from build123d import *

# Parameters (mm, degrees)
SKETCH1_R                = 2
BOSS_EXTRUDE2_DEPTH      = 5
BOSS_EXTRUDE3_DEPTH      = 9
BOSS_EXTRUDE3_DEPTH_BACK = 14
SKETCH3_W                = 35
SKETCH3_H                = 50
SKETCH4_W                = 13
SKETCH4_H                = 40
CUT_EXTRUDE1_DEPTH       = 194.703381488
SKETCH5_R                = 4.35
CUT_EXTRUDE2_DEPTH       = 194.053917795
CUT_EXTRUDE3_DEPTH       = 193.189529309
FILLET14_R               = 15
FILLET15_R               = 15
FILLET16_R               = 15
FILLET17_R               = 15
FILLET18_R               = 5
FILLET19_R               = 5
FILLET20_R               = 5
FILLET21_R               = 5
FILLET22_R               = 3
FILLET23_R               = 3
FILLET24_R               = 3
FILLET25_R               = 3
SKETCH7_R                = 4
CUT_EXTRUDE4_DEPTH       = 193.189529428


with BuildPart() as part:
    # Sketch1 → Boss-Extrude2 (new body)
    with BuildSketch(Plane.XY):
        with BuildLine():
            Line((-9.685672515, -15), (-9.685672515, 190))
            Line((-9.685672515, 190), (25.314327485, 190))
            Line((25.314327485, 190), (25.314327485, -15))
            ThreePointArc((25.314327485, -15), (7.814327485, -32.5), (-9.685672515, -15))
        make_face()
        with Locations((19.814327485, -15)):
            Circle(SKETCH1_R, mode=Mode.SUBTRACT)
        with Locations((7.814327485, -27)):
            Circle(SKETCH1_R, mode=Mode.SUBTRACT)
        with Locations((-4.185672515, -15)):
            Circle(SKETCH1_R, mode=Mode.SUBTRACT)
        with Locations((7.814327485, -3)):
            Circle(SKETCH1_R, mode=Mode.SUBTRACT)
    extrude(amount=BOSS_EXTRUDE2_DEPTH)

    # Sketch3 → Boss-Extrude3 (add, two sides: drawn at the far end of the back side and taken through both)
    with BuildSketch(Plane.XY.offset(5).offset(-BOSS_EXTRUDE3_DEPTH_BACK)):
        with Locations((7.814327485, 165)):
            Rectangle(SKETCH3_W, SKETCH3_H)
    extrude(amount=BOSS_EXTRUDE3_DEPTH + BOSS_EXTRUDE3_DEPTH_BACK)

    # Sketch4 → Cut-Extrude1 (cut, through all)
    with BuildSketch(Plane(origin=(25.314327485, 0, 0), x_dir=(0, 0, -1), z_dir=(1, 0, 0))):
        with Locations((-2.5, 170)):
            Rectangle(SKETCH4_W, SKETCH4_H)
    extrude(amount=-CUT_EXTRUDE1_DEPTH, mode=Mode.SUBTRACT)

    # Sketch5 → Cut-Extrude2 (cut, through all)
    with BuildSketch(Plane.XY.offset(14)):
        with Locations((7.814327485, 176)):
            Circle(SKETCH5_R)
    extrude(amount=-CUT_EXTRUDE2_DEPTH, mode=Mode.SUBTRACT)

    # Sketch6 → Cut-Extrude3 (cut, through all)
    with BuildSketch(Plane.XY.offset(5)):
        with BuildLine():
            Line((15.314327485, 118), (15.314327485, 78))
            ThreePointArc((15.314327485, 78), (7.814327485, 70.5), (0.314327485, 78))
            Line((0.314327485, 78), (0.314327485, 118))
            ThreePointArc((0.314327485, 118), (7.814327485, 125.5), (15.314327485, 118))
        make_face()
        with BuildLine():
            Line((15.314327485, 53), (15.314327485, 13))
            ThreePointArc((15.314327485, 13), (7.814327485, 5.5), (0.314327485, 13))
            Line((0.314327485, 13), (0.314327485, 53))
            ThreePointArc((0.314327485, 53), (7.814327485, 60.5), (15.314327485, 53))
        make_face()
    extrude(amount=-CUT_EXTRUDE3_DEPTH, mode=Mode.SUBTRACT)

    # Fillet14
    fillet14_edges = [part.edges().sort_by_distance(p)[0] for p in [
        (25.314327485, 190, 11.5),
    ]]
    fillet(fillet14_edges, radius=FILLET14_R)

    # Fillet15
    fillet15_edges = [part.edges().sort_by_distance(p)[0] for p in [
        (-9.685672515, 190, 11.5),
    ]]
    fillet(fillet15_edges, radius=FILLET15_R)

    # Fillet16
    fillet16_edges = [part.edges().sort_by_distance(p)[0] for p in [
        (-9.685672515, 190, -6.5),
    ]]
    fillet(fillet16_edges, radius=FILLET16_R)

    # Fillet17
    fillet17_edges = [part.edges().sort_by_distance(p)[0] for p in [
        (25.314327485, 190, -6.5),
    ]]
    fillet(fillet17_edges, radius=FILLET17_R)

    # Fillet18
    fillet18_edges = [part.edges().sort_by_distance(p)[0] for p in [
        (7.814327485, 140, 5),
    ]]
    fillet(fillet18_edges, radius=FILLET18_R)

    # Fillet19
    fillet19_edges = [part.edges().sort_by_distance(p)[0] for p in [
        (7.814327485, 140, 0),
    ]]
    fillet(fillet19_edges, radius=FILLET19_R)

    # Fillet20
    fillet20_edges = [part.edges().sort_by_distance(p)[0] for p in [
        (7.814327485, 140, -9),
    ]]
    fillet(fillet20_edges, radius=FILLET20_R)

    # Fillet21
    fillet21_edges = [part.edges().sort_by_distance(p)[0] for p in [
        (7.814327485, 140, 14),
    ]]
    fillet(fillet21_edges, radius=FILLET21_R)

    # Fillet22
    fillet22_edges = [part.edges().sort_by_distance(p)[0] for p in [
        (0.314327485, 98, 0),
        (7.814327485, 70.5, 0),
        (15.314327485, 98, 0),
        (7.814327485, 125.5, 0),
    ]]
    fillet(fillet22_edges, radius=FILLET22_R)

    # Fillet23
    # the kernel refuses this fillet: 3 mm, written as the material it takes off along each edge
    with BuildSketch(Plane(origin=(15.314327485, 118, 5), x_dir=(0, 0, -1), z_dir=(0, -1, 0)), Plane(origin=(0.314327485, 78, 5), x_dir=(0, 0, -1), z_dir=(0, 1, 0))) as fillet23_piece_1:
        with BuildLine():
            CenterArc((3, 2.828427125), FILLET23_R, 180, 70.528779366)
            Line((0, 2.828427125), (-0.06, 2.828427125))
            Line((-0.06, 2.828427125), (-0.06, 0))
            Line((-0.06, 0), (0, -0.06))
            ThreePointArc((0, -0.06), (1, -0.06), (1.98, -0.056568542))
            Line((1.98, -0.056568542), (2, 0))
        make_face()
    extrude(amount=40, mode=Mode.SUBTRACT)
    with BuildSketch(Plane(origin=(7.814327485, 78, 5), x_dir=(1, 0, 0), z_dir=(0, 1, 0))) as fillet23_piece_2:
        with BuildLine():
            CenterArc((10.328427125, 3), FILLET23_R, 199.471220634, 70.528779366)
            Line((10.328427125, 0), (10.328427125, -0.06))
            Line((10.328427125, -0.06), (7.5, -0.06))
            Line((7.5, -0.06), (7.44, 0))
            ThreePointArc((7.44, 0), (7.44, 1), (7.443431458, 1.98))
            Line((7.443431458, 1.98), (7.5, 2))
        make_face()
    revolve(axis=Axis((7.814327485, 78, 5), (0, 0, -1)), revolution_arc=180, mode=Mode.SUBTRACT)
    with BuildSketch(Plane(origin=(7.814327485, 118, 5), x_dir=(-1, 0, 0), z_dir=(0, -1, 0))) as fillet23_piece_3:
        with BuildLine():
            CenterArc((10.328427125, 3), FILLET23_R, 199.471220634, 70.528779366)
            Line((10.328427125, 0), (10.328427125, -0.06))
            Line((10.328427125, -0.06), (7.5, -0.06))
            Line((7.5, -0.06), (7.44, 0))
            ThreePointArc((7.44, 0), (7.44, 1), (7.443431458, 1.98))
            Line((7.443431458, 1.98), (7.5, 2))
        make_face()
    revolve(axis=Axis((7.814327485, 118, 5), (0, 0, -1)), revolution_arc=180, mode=Mode.SUBTRACT)

    # Fillet24
    fillet24_edges = [part.edges().sort_by_distance(p)[0] for p in [
        (0.314327485, 33, 0),
        (7.814327485, 5.5, 0),
        (15.314327485, 33, 0),
        (7.814327485, 60.5, 0),
    ]]
    fillet(fillet24_edges, radius=FILLET24_R)

    # Fillet25
    # the kernel refuses this fillet: 3 mm, written as the material it takes off along each edge
    with BuildSketch(Plane(origin=(15.314327485, 53, 5), x_dir=(0, 0, -1), z_dir=(0, -1, 0)), Plane(origin=(0.314327485, 13, 5), x_dir=(0, 0, -1), z_dir=(0, 1, 0))) as fillet25_piece_1:
        with BuildLine():
            CenterArc((3, 2.828427125), FILLET25_R, 180, 70.528779366)
            Line((0, 2.828427125), (-0.06, 2.828427125))
            Line((-0.06, 2.828427125), (-0.06, 0))
            Line((-0.06, 0), (0, -0.06))
            ThreePointArc((0, -0.06), (1, -0.06), (1.98, -0.056568542))
            Line((1.98, -0.056568542), (2, 0))
        make_face()
    extrude(amount=40, mode=Mode.SUBTRACT)
    with BuildSketch(Plane(origin=(7.814327485, 13, 5), x_dir=(1, 0, 0), z_dir=(0, 1, 0))) as fillet25_piece_2:
        with BuildLine():
            CenterArc((10.328427125, 3), FILLET25_R, 199.471220634, 70.528779366)
            Line((10.328427125, 0), (10.328427125, -0.06))
            Line((10.328427125, -0.06), (7.5, -0.06))
            Line((7.5, -0.06), (7.44, 0))
            ThreePointArc((7.44, 0), (7.44, 1), (7.443431458, 1.98))
            Line((7.443431458, 1.98), (7.5, 2))
        make_face()
    revolve(axis=Axis((7.814327485, 13, 5), (0, 0, -1)), revolution_arc=180, mode=Mode.SUBTRACT)
    with BuildSketch(Plane(origin=(7.814327485, 53, 5), x_dir=(-1, 0, 0), z_dir=(0, -1, 0))) as fillet25_piece_3:
        with BuildLine():
            CenterArc((10.328427125, 3), FILLET25_R, 199.471220634, 70.528779366)
            Line((10.328427125, 0), (10.328427125, -0.06))
            Line((10.328427125, -0.06), (7.5, -0.06))
            Line((7.5, -0.06), (7.44, 0))
            ThreePointArc((7.44, 0), (7.44, 1), (7.443431458, 1.98))
            Line((7.443431458, 1.98), (7.5, 2))
        make_face()
    revolve(axis=Axis((7.814327485, 53, 5), (0, 0, -1)), revolution_arc=180, mode=Mode.SUBTRACT)

    # Sketch7 → Cut-Extrude4 (cut, through all)
    with BuildSketch(Plane.XY.offset(5)):
        with Locations((7.814327485, -15)):
            Circle(SKETCH7_R)
    extrude(amount=-CUT_EXTRUDE4_DEPTH, mode=Mode.SUBTRACT)


solid = part.part
Check sheet for the modelled part. Datum: model origin and axes. Units: mm. A direction names the side the tool comes from. Round coordinates to 2 decimals unless told otherwise and drop trailing zeros. Loops run counter-clockwise (first coordinate to the right, second up) from the corner with the lowest first, then second, coordinate; pieces in that order, holes last. Notation, with made-up numbers: (26.25, 57) -> (68.25, 57) arc R9 cw to (68.25, 72) -> close; hole circle Ø10 at (38.5, 48). An arc over 180 degrees is marked (long way). Put each result on its own line as item: value. Start each with the question number.
1. Draft check along Y on faces 1 (the face through (-5.2, 185.7, 11.5)), 2 (the face through (-9.686, 101, 2)), 3 (the face through (6.23, -4.22, 2.46)), 4 (the face through (11.63, -13.8, 2.54)). Enter one of: +Y half, -Y half, draft (parallel to the pull), parting line (faces both ways), or undercut.
2. Section check C-C (y = 156). Enter the section's corners in (x, z), plus the area to 3 significant figures.
3. Section check B-B (y = 46). Enter the section's corners in (x, z).
4. Access from +Z, -Z, +X, -X, +Y, -Y to the whole of each face (thin tool, end or side, straight path). Record for faces 5 (the face through (6.871, 171.753, 11.535)), 6 (the face through (8, 170, 9)).
5. Gauge pin test, flat ends, axial feed: pin 1 (6.5 mm diameter, centred on x = 19.81, y = -15, fed in from -Z); pin 2 (5 mm diameter, centred on x = 17, z = 11.5, fed in from +Y); pin 3 (10 mm diameter, centred on x = 1.5, y = 54.5, fed in from +Z); pin 4 (7 mm diameter, centred on x = 7.81, y = 176, fed in from +Z). Record the tip position at first contact, or that the pin passes through.
6. Section check A-A (y = -3). Enter the section's corners in (x, z).
7. Scan lines: probe 1 along Z at (x, y) = (13.5, 169); probe 2 along Y at (x, z) = (5.5, 3.75); probe 3 along Y at (x, z) = (6, 0.75). Record each from-to range of solid material in increasing order.
Findings:
1. face 1: +Y half
1. face 2: draft
1. face 3: undercut
1. face 4: undercut
2. outline: (-9.69, -9) -> (25.31, -9) -> (25.31, -4) -> (-9.69, -4) -> close; (-9.69, 9) -> (25.31, 9) -> (25.31, 14) -> (-9.69, 14) -> close
2. area: 350 mm^2
3. outline: (-9.69, 0) -> (-2.69, 0) arc R3 ccw to (0.31, 3) arc R3 ccw to (-2.51, 5) -> (-9.69, 5) -> close; (15.31, 3) arc R3 ccw to (18.31, 0) -> (25.31, 0) -> (25.31, 5) -> (18.14, 5) arc R3 ccw to start
4. face 5: +Z, -Z
4. face 6: +X, -X, +Y
5. pin 1: stops at z = 0
5. pin 2: stops at y = 189.4
5. pin 3: stops at z = 5
5. pin 4: passes through
6. outline: (-9.69, 0) -> (5.81, 0) -> (5.81, 5) -> (-9.69, 5) -> close; (9.81, 0) -> (25.31, 0) -> (25.31, 5) -> (9.81, 5) -> close
7. probe 1: z = -9 to -4, 9 to 14
7. probe 2: y = -32.35 to -18.26, -11.74 to 5.46, 60.54 to 70.46, 125.54 to 150
7. probe 3: y = -32.41 to -27.84, -26.16 to -18.56, -11.44 to -3.84, -2.16 to 4.68, 61.32 to 69.68, 126.32 to 150
